Input: part model. Units: mm. Frame: model coordinates. A direction names the side the tool comes from. Round coordinates to 2 decimals unless told otherwise and drop trailing zeros. Loops run counter-clockwise (first coordinate to the right, second up) from the corner with the lowest first, then second, coordinate; pieces in that order, holes last.
(1) First-contact query: pin 1 Ø1.9 at (x, z) = (-120.5, 3) entering from -Y. Flat tip, straight axial feed; report the tip coordinate or a pass-through.
(2) Draft query along Y for faces 3 (the face through (-298.45, 107, 3)), 4 (the face through (-147, 0, 3)), 5 (the face through (-323.85, 106, 3)). Return one class per face: released by +Y, released by -Y, zero draft, split by the parting line, or undercut.
(3) Cut plane B-B, the plane y = 132. Output: boundary loops of the cut face in (x, z).
(4) Access query for faces 1 (the face through (25.4, 109, 3)), 2 (the face through (0, 109, 3)). Directions: +Z, -Z, +X, -X, +Y, -Y. A direction counts if a zero-diameter tool reaches every point of the face in a straight line with its end or side. Return the directions, or none.
(5) Line query: line 1 (X direction, y = 30, z = 1.5); line 2 (Y direction, x = -97, z = 1). Output: solid intervals per line, ascending.
(6) Cut plane C-C, the plane z = 2.25. Output: boundary loops of the cut face in (x, y).
(7) Cut plane A-A, the plane x = -263. Output: boundary loops of the cut face in (y, z), and give its area (3 significant figures).
Autodesk Inventor part; units mm, degrees
ref_plane "YZ Plane" through (0, 0, 0) normal (1, 0, 0) x (0, 1, 0)
ref_plane "XZ Plane" through (0, 0, 0) normal (0, 1, 0) x (-1, 0, 0)
ref_plane "XY Plane" through (0, 0, 0) normal (0, 0, 1) x (1, 0, 0)
sketch "Sketch1" plane through (0, 0, 0) normal (0, 0, 1) x (1, 0, 0)
  line L0 (0, 0) -> (0, 25.4)
  line L1 (0, 25.4) -> (-298.45, 25.4)
  line L2 (-298.45, 0) -> (-298.45, 25.4)
  line L3 (0, 0) -> (-298.45, 0)
  line L4 (-323.85, 0) -> (-298.45, 0)
  line L5 (-298.45, 0) -> (-298.45, 215.9)
  line L6 (-323.85, 215.9) -> (-298.45, 215.9)
  line L7 (-323.85, 0) -> (-323.85, 215.9)
  line L8 (-298.45, 215.9) -> (-298.45, 190.5)
  line L9 (-298.45, 190.5) -> (0, 190.5)
  line L10 (0, 215.9) -> (0, 190.5)
  line L11 (-298.45, 215.9) -> (0, 215.9)
  line L12 (25.4, 215.9) -> (0, 215.9)
  line L13 (0, 215.9) -> (0, 0)
  line L14 (25.4, 0) -> (0, 0)
  line L15 (25.4, 215.9) -> (25.4, 0)
  line L16 (-323.85, 0) -> (25.4, 0)
  line L17 (25.4, 0) -> (25.4, 215.9)
  line L18 (25.4, 215.9) -> (-323.85, 215.9)
  line L19 (-323.85, 215.9) -> (-323.85, 0)
  line L20 (0, 25.4) -> (-298.45, 25.4)
  line L21 (-298.45, 25.4) -> (-298.45, 190.5)
  line L22 (-298.45, 190.5) -> (0, 190.5)
  line L23 (0, 190.5) -> (0, 25.4)
  dimension "d0" = 25.4
  dimension "d1" = 25.4
  dimension "d2" = 215.9
  dimension "d3" = 25.4
  dimension "d4" = 25.4
extrude "Extrusion1" add sketch "Sketch1" along normal blind 6.35 contours L3 L2 L1 L0 | L0 L13 L10 L12 L15 L14 | L4 L7 L6 L5 L2 | L9 L5 L11 L10
properties part number "Velcro strip"
Reported:
1. pin 1: stops at y = 0
2. face 3: undercut
2. face 4: released by -Y
2. face 5: zero draft
3. outline: (-323.85, 0) - (-298.45, 0) - (-298.45, 6.35) - (-323.85, 6.35) - close; (0, 0) - (25.4, 0) - (25.4, 6.35) - (0, 6.35) - close
4. face 1: +Z, -Z, +X, +Y, -Y
4. face 2: +Z, -Z
5. line 1: x = -323.85 to -298.45, 0 to 25.4
5. line 2: y = 0 to 25.4, 190.5 to 215.9
6. outline: (-323.85, 0) - (25.4, 0) - (25.4, 215.9) - (-323.85, 215.9) - close; hole (-298.45, 25.4) - (0, 25.4) - (0, 190.5) - (-298.45, 190.5) - close
7. outline: (0, 0) - (25.4, 0) - (25.4, 6.35) - (0, 6.35) - close; (190.5, 0) - (215.9, 0) - (215.9, 6.35) - (190.5, 6.35) - close
7. area: 323 mm2
